from build123d import *

# Parameters (mm, degrees)
SKETCH1_R           = 120
BOSS_EXTRUDE1_DEPTH = 30
BOSS_EXTRUDE2_DEPTH = 60
CIRPATTERN1_COUNT   = 16
SKETCH3_R           = 80
BOSS_EXTRUDE3_DEPTH = 72
CUT_EXTRUDE1_DEPTH  = 249.179654279


with BuildPart() as part:
    # Sketch1 → Boss-Extrude1 (new, symmetric)
    with BuildSketch(Plane(origin=(0, 0, 0), x_dir=(0, 0, -1), z_dir=(1, 0, 0))):
        Circle(SKETCH1_R)
    extrude(amount=BOSS_EXTRUDE1_DEPTH, both=True)

    # Sketch2 → Boss-Extrude2 (add)
    with BuildSketch(Plane(origin=(30, 0, 0), x_dir=(0, 0, -1), z_dir=(1, 0, 0))):
        with BuildLine():
            Line((-6, 142.928549979), (6, 142.928549979))
            ThreePointArc((6, 142.928549979), (12.813200818, 131.684050319), (16, 118.928549979))
            ThreePointArc((16, 118.928549979), (0, -120), (-16, 118.928549979))
            ThreePointArc((-16, 118.928549979), (-12.813200818, 131.684050319), (-6, 142.928549979))
        make_face()
    boss_extrude2 = extrude(amount=-BOSS_EXTRUDE2_DEPTH)

    # CirPattern1: Boss-Extrude2 ×16 about axis
    cirpattern1_axis = Axis((0, 0, 0), (1, 0, 0))
    for i in range(1, CIRPATTERN1_COUNT):
        add(boss_extrude2.rotate(cirpattern1_axis, i * 360 / CIRPATTERN1_COUNT))

    # Sketch3 → Boss-Extrude3 (add, symmetric)
    with BuildSketch(Plane(origin=(0, 0, 0), x_dir=(0, 0, -1), z_dir=(1, 0, 0))):
        Circle(SKETCH3_R)
    extrude(amount=BOSS_EXTRUDE3_DEPTH, both=True)

    # Sketch4 → Cut-Extrude1 (cut, through all)
    with BuildSketch(Plane(origin=(72, 0, 0), x_dir=(0, 0, -1), z_dir=(1, 0, 0))):
        with BuildLine():
            Line((-16, 60), (16, 60))
            Line((16, 60), (16, 47.370877129))
            ThreePointArc((16, 47.370877129), (0, -50), (-16, 47.370877129))
            Line((-16, 47.370877129), (-16, 60))
        make_face()
    extrude(amount=-CUT_EXTRUDE1_DEPTH, mode=Mode.SUBTRACT)


solid = part.part
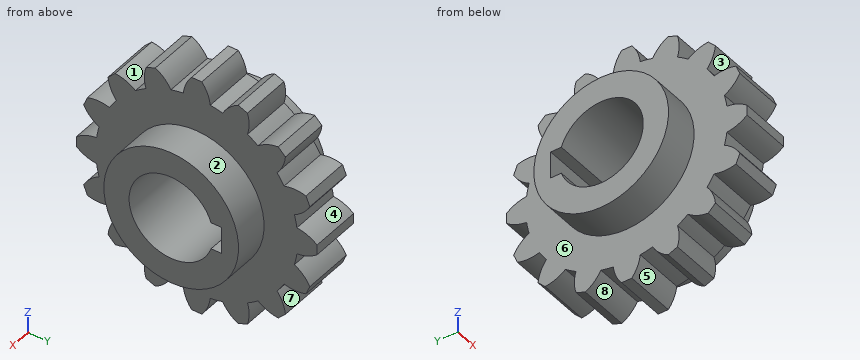
Can you work these out from the model? Positions are in its coordinate system, mm. Face numbers are marked on the shaded views. A direction names the side the tool comes from. Coordinates: 2 decimals unless noted, no trailing zeros. Write each loop counter-clockwise with the first axis right and the second up, starting at its lowest first coordinate (ties: lowest second). Pieces come first, ordered by that corner, then holes. Notation, with made-up numbers: (39, 32.5) -> (81, 32.5) arc R31 ccw to (81, 61.5) -> close; hole circle Ø7 at (-40, 61.5). An arc over 180 degrees is marked (long way). Answer as CSV lines item,"result".
1) If we section it at B-B on z = 0: Please give me the cut outline in (x, y).
Check result:
outline,"(-72, -80) -> (-30, -80) -> (-30, -142.93) -> (30, -142.93) -> (30, -80) -> (72, -80) -> (72, -50) -> (-72, -50) -> close; (-72, 60) -> (72, 60) -> (72, 80) -> (30, 80) -> (30, 142.93) -> (-30, 142.93) -> (-30, 80) -> (-72, 80) -> close"
2) Will these pins go through, and if not, where does the flat tip stop? P1, Ø12, axis at x = -57.5, y = 41, coming from the -Z side; P2, Ø4, axis at x = -34, y = 55.5, coming from the -Z side; P3, Ø3, axis at y = -34.5, z = 92.5, coming from the +X side.
Check result:
P1,"z = -71.94"
P2,"z = -59.48"
P3,"x = 30"
3) If we section it at C-C on x = -47: Please give me the cut outline in (y, z), then the cut area to 3 significant figures.
Check result:
outline,"circle Ø160 at (0, 0); hole (47.37, -16) -> (60, -16) -> (60, 16) -> (47.37, 16) arc R50 ccw (long way) to start"
area,"11,900 mm²"
4) On a 3-axis mill with a long thin cutter (end or side, diameter ignored), from which of +Z, -Z, +X, -X, +Y, -Y can I reach the whole of each face in a straight line? I mean the marked faces 1, 2, 3, 4 and 5. Say none if no direction works.
Check result:
face 1,"+Z, +X, -X"
face 2,"+X"
face 3,"+X, -X, -Y"
face 4,"+X, -X, +Y"
face 5,"-Z, +X, -X"
5) If we section it at A-A on y = 0: Please give me the cut outline in (x, z), then the cut area to 3 significant figures.
Check result:
outline,"(-72, -80) -> (-30, -80) -> (-30, -142.93) -> (30, -142.93) -> (30, -80) -> (72, -80) -> (72, -50) -> (-72, -50) -> close; (-72, 50) -> (72, 50) -> (72, 80) -> (30, 80) -> (30, 142.93) -> (-30, 142.93) -> (-30, 80) -> (-72, 80) -> close"
area,"16,200 mm²"
6) If I drill on line 1 (Y direction, x = 30.5, z = 0); line 2 (Y direction, x = 15.5, z = 0); line 3 (Y direction, x = 22.5, z = 125), over which ranges is the centre line in solid material (lowest first)? Write a range as from..to.
Check result:
line 1,"-80..-50, 60..80"
line 2,"-142.93..-50, 60..142.93"
line 3,"-61.43..-37.06, -14.99..14.99, 37.06..61.43"
7) If we mould it in two halves opening along Y, with no side actions, what happens to the marked faces 6, 7 and 8? For each: +Y half, -Y half, draft (parallel to the pull), parting line (faces both ways), or undercut.
Check result:
face 6,"draft"
face 7,"+Y half"
face 8,"undercut"
